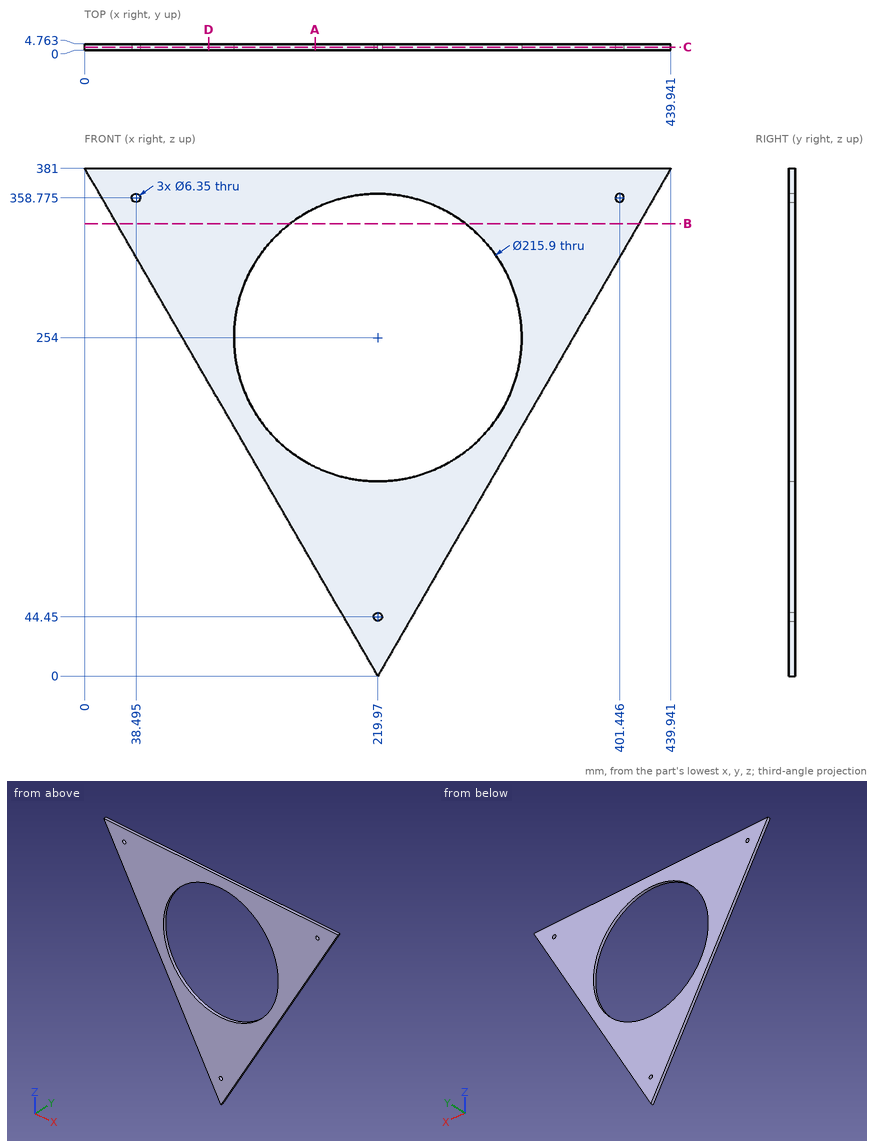
Study the drawing (mm; zero at the part's minimum x, y, z) and answer. Round coordinates to 2 decimals unless told otherwise and drop trailing zeros. Write each loop counter-clockwise with the first axis right and the second up, starting at its lowest first coordinate (ties: lowest second). Pieces come first, ordered by that corner, then holes.
1) A cutting plane is placed at B-B (z = 339.5). Give the vertices of the cut face in (x, y), plus the area to 3 significant figures.
2) Given pin 1 Ø1 at (y, z) = (1, 78) entering from -X; pin 2 Ø1.5 at (y, z) = (1.5, 332.5) entering from +X, each flat-ended and moving along its own axis, determine where each tip first touches the part or whether it passes through.
3) A cutting plane is placed at C-C (y = 2.4). Give the number of separate pieces and of enclosed holes in the cut face, plus the area to 3 significant figures.
4) A cutting plane is placed at D-D (x = 93). Give the vertices of the cut face in (y, z), plus the area to 3 significant figures.
5) Straight lines are drawn through the part: line 1 (Z direction, x = 39, y = 1.45); line 2 (Z direction, x = 224, y = 0.5) (1 decimal); line 3 (X direction, y = 0.55, z = 274.5) (1 decimal). For each, find the intervals that lie inside material, in ascending order.
6) A cutting plane is placed at A-A (x = 173). Give the vertices of the cut face in (y, z) (1 decimal).
Completed:
1. outline: (23.96, 0) - (154.07, 0) - (154.07, 4.76) - (23.96, 4.76) - close; (285.87, 0) - (415.98, 0) - (415.98, 4.76) - (285.87, 4.76) - close
1. area: 1,240 mm2
2. pin 1: stops at x = 174.65
2. pin 2: stops at x = 412.37
3. separate pieces: 1
3. enclosed holes: 4
3. area: 47,100 mm2
4. outline: (0, 219.92) - (4.76, 219.92) - (4.76, 381) - (0, 381) - close
4. area: 767 mm2
5. line 1: z = 313.45 to 355.64, 361.91 to 381
5. line 2: z = 7 to 146.1, 361.9 to 381
5. line 3: x = 61.5 to 114, 326 to 378.5
6. outline: (0, 81.4) - (4.8, 81.4) - (4.8, 156.8) - (0, 156.8) - close; (0, 351.2) - (4.8, 351.2) - (4.8, 381) - (0, 381) - close
